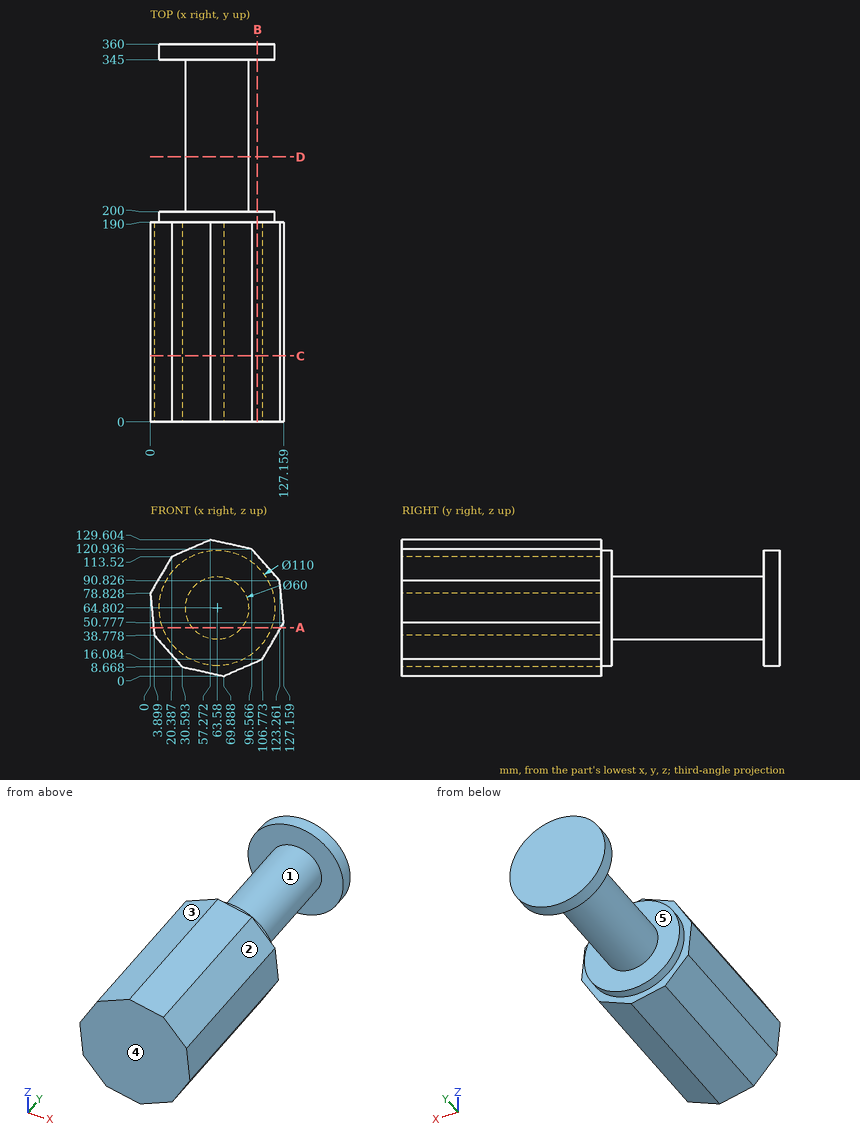
Here's the drawing with two shaded views (mm, measured from the low corner). I have some questions. A direction names the side the tool comes from. Give positions to 0.01 mm unless a question says otherwise; leave off trailing zeros. Order: outer loops, then holes, each group sorted by start corner. A loop starts at its lowest first (then second) coordinate and runs counter-clockwise, first axis right, second up. Notation, with made-up numbers: M 3.25,16 L 52.25,16 A14 ccw 52.25,42 Z; hole C -7.75,52 d9. An arc over 180 degrees is marked long. One line per item, written item: value.
1) Please list where these lines run through material, in increasing order: line 1 along Y through (x, z) = (28, 62.5); line 2 along Y through (x, z) = (89, 120); line 3 along X through (y, z) = (158, 40.5).
Answer sheet:
line 1: y = 0 to 200, 345 to 360
line 2: y = 0 to 190
line 3: x = 3.73 to 121.12
2) We'd pull the mould along Y, two halves only. Please class the marked faces 3, 4 and 5: released by +Y, released by -Y, zero draft, split by the parting line, or undercut.
Answer sheet:
face 3: zero draft
face 4: released by -Y
face 5: undercut
3) I want a section at B-B, the plane x = 102. List the corners of the cut face in (y, z) for me, plus the area to 3 significant figures.
Answer sheet:
outline: M 0,14 L 190,14 L 190,25.45 L 200,25.45 L 200,104.16 L 190,104.16 L 190,114.81 L 0,114.81 Z; M 345,25.45 L 360,25.45 L 360,104.16 L 345,104.16 Z
area: 21,100 mm^2
4) I want a section at A-A, the plane z = 46. List the corners of the cut face in (x, y) for me (1 decimal).
Answer sheet:
outline: M 3.2,0 L 124.4,0 L 124.4,190 L 115.3,190 L 115.3,200 L 87,200 L 87,345 L 115.3,345 L 115.3,360 L 11.9,360 L 11.9,345 L 40.2,345 L 40.2,200 L 11.9,200 L 11.9,190 L 3.2,190 Z
5) For P1, Ø1, axis at y = 185.5, z = 69.5, coming from the +X side (1 decimal); P2, Ø6, axis at x = 73, y = 166, coming from the +Z side; P3, Ø6, axis at y = 195.5, z = 98.5, coming from the +X side (1 decimal); P4, Ø2, axis at x = 23.5, z = 26, coming from the -Y side, each with a flat end and sliding along its axis, tell me the tip position at first contact or that it passes through.
Answer sheet:
P1: stops at x = 125.4
P2: stops at z = 126.8
P3: stops at x = 109.2
P4: stops at y = 0
6) I want a section at C-C, the plane y = 63. List the corners of the cut face in (x, z) for me (1 decimal).
Answer sheet:
outline: M 0,78.8 L 3.9,38.8 L 30.6,8.7 L 69.9,0 L 106.8,16.1 L 127.2,50.8 L 123.3,90.8 L 96.6,120.9 L 57.3,129.6 L 20.4,113.5 Z
7) I want a section at D-D, the plane y = 252.5. List the corners of the cut face in (x, z) for me, plus the area to 3 significant figures.
Answer sheet:
outline: C 63.58,64.8 d60
area: 2,830 mm^2
8) On a 3-axis mill with a long thin cutter (end or side, diameter ignored), from which of +Z, -Z, +X, -X, +Y, -Y can I reach the whole of each face in a straight line? I mean the marked faces 1 and 2. Say none if no direction works.
Answer sheet:
face 1: none
face 2: +Z, +X, +Y, -Y
